Check sheet for the modelled part. Datum: model origin and axes. Units: mm. Face numbers are marked on the shaded views. A direction names the side the tool comes from. Give positions to 0.01 mm unless a question says otherwise; leave off trailing zeros. Write each loop counter-clockwise with the first axis right and the second up, starting at its lowest first coordinate (ties: lowest second). Pieces come first, ordered by that corner, then holes. Notation, with made-up numbers: M 24.25,-38 L 28.25,-38 A20 ccw 28.25,-20 Z; hole C 77,84.5 d11. An arc over 180 degrees is marked long. Use CSV: the item, a comma, the result in double quotes. Start each with the question number.
1. Access from +Z, -Z, +X, -X, +Y, -Y to the whole of each face (thin tool, end or side, straight path). Record for the marked faces 1, 2, 3 and 4.
2. Cross-section at C-C, the plane x = 4. Enter the section's corners in (y, z), and give its area (3 significant figures).
3. Cross-section at A-A, the plane y = 25.5. Enter the section's corners in (x, z).
4. Cross-section at D-D, the plane y = 66.5. Enter the section's corners in (x, z).
5. Scan lines: line 1 (Y direction, x = -7.25, z = 0.75); line 2 (Y direction, x = -0.5, z = -5.5); line 3 (X direction, y = 29.5, z = -6.5). Record each from-to range of solid material in increasing order.
6. Depth check by flat-ended pin: P1, Ø2, axis at y = 16, z = 1.5, coming from the -X side; P2, Ø6, axis at y = 34.5, z = 0.5, coming from the +X side; P3, Ø2, axis at y = 17, z = -0.5, coming from the +X side. Enter the tip coordinate at first touch or a pass-through.
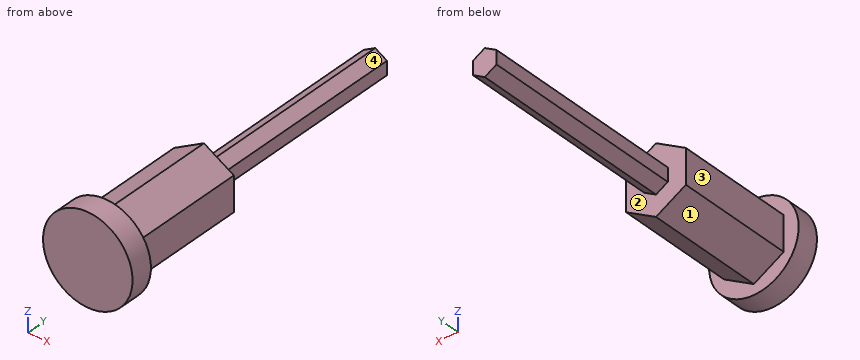
Autodesk Inventor part; units mm, degrees
ref_plane "YZ Plane" through (0, 0, 0) normal (1, 0, 0) x (0, 1, 0)
ref_plane "XZ Plane" through (0, 0, 0) normal (0, 1, 0) x (-1, 0, 0)
ref_plane "XY Plane" through (0, 0, 0) normal (0, 0, 1) x (1, 0, 0)
sketch "Sketch1" plane through (0, 0, 0) normal (0, 1, 0) x (-1, 0, 0)
  circle A0 centre (0, 0) radius 9.525
  dimension "d0" = 19.05
extrude "Extrusion1" add sketch "Sketch1" along normal blind 4.7625
sketch "Sketch2" plane through (0, 4.7625, 0) normal (0, 1, 0) x (1, 0, 0)
  line L0 (0, -7.3323) -> (-6.35, -3.6662)
  line L1 (-6.35, -3.6662) -> (-6.35, 3.6662)
  line L2 (-6.35, 3.6662) -> (0, 7.3323)
  line L3 (0, 7.3323) -> (6.35, 3.6662)
  line L4 (6.35, 3.6662) -> (6.35, -3.6662)
  line L5 (6.35, -3.6662) -> (0, -7.3323)
  line L6 (0, 0) -> (0, -9.525)
  circle A0 centre (0, 0) radius 9.525
  dimension "d3" = 12.7
extrude "Extrusion2" add sketch "Sketch2" along normal blind 25.4 contours L0 L1 L2 L3 L4 L5
sketch "Sketch3" plane through (0, 30.1625, 0) normal (0, 1, 0) x (1, 0, 0)
  line L0 (0, 2.8868) -> (2.5, 1.4434)
  line L1 (2.5, 1.4434) -> (2.5, -1.4434)
  line L2 (2.5, -1.4434) -> (0, -2.8868)
  line L3 (0, -2.8868) -> (-2.5, -1.4434)
  line L4 (-2.5, -1.4434) -> (-2.5, 1.4434)
  line L5 (-2.5, 1.4434) -> (0, 2.8868)
  line L6 (-6.35, -3.6662) -> (0, -7.3323)
  line L7 (0, 0) -> (0, -7.3323)
  dimension "d6" = 5
extrude "Extrusion3" add sketch "Sketch3" along normal blind 44.45
properties part number "0.5in hex to 5mm hex"
Worked answers:
1,face 1,"-Z, -X, +Y"
1,face 2,"+Y"
1,face 3,"+Z, -Z, -X, +Y"
1,face 4,"+Z, +X, +Y"
2,outline,"M 0,-8.64 L 4.76,-8.64 L 4.76,-5.02 L 30.16,-5.02 L 30.16,5.02 L 4.76,5.02 L 4.76,8.64 L 0,8.64 Z"
2,area,"338 mm^2"
3,outline,"M -6.35,-3.67 L 0,-7.33 L 6.35,-3.67 L 6.35,3.67 L 0,7.33 L -6.35,3.67 Z"
4,outline,"M -2.5,-1.44 L 0,-2.89 L 2.5,-1.44 L 2.5,1.44 L 0,2.89 L -2.5,1.44 Z"
5,line 1,"y = 0 to 4.76"
5,line 2,"y = 0 to 30.16"
5,line 3,"x = -1.44 to 1.44"
6,P1,"stops at x = -6.35"
6,P2,"stops at x = 2.5"
6,P3,"stops at x = 6.35"
